Design review of the part shown in the three views and the two pictorial views. Dimensions are in mm from the part's minimum x, y and z. A direction names the side the tool comes from. Coordinates: 2 decimals unless noted, no trailing zeros. Order: outer loops, then holes, each group sorted by start corner. A loop starts at its lowest first (then second) coordinate and runs counter-clockwise, first axis right, second up. Notation, with made-up numbers: (26.25, 88) -> (75.25, 88) arc R36 ccw to (75.25, 127) -> close; hole circle Ø4 at (49.25, -1.5). An arc over 180 degrees is marked (long way). Answer as a JSON object with one key per item and string values. Group by question number.
1) Add section B-B, the plane z = 10.5. Write out the cut boundary in (x, y), then the cut area to 3 significant figures.
2) Add section D-D, the plane y = 40. Write out the cut boundary in (x, z), then the cut area to 3 significant figures.
3) Add section C-C, the plane z = 34. Write out the cut boundary in (x, y), then the cut area to 3 significant figures.
4) Machinability: for the marked faces 1 and 2, which of the approach directions +Z, -Z, +X, -X, +Y, -Y give a long, thin tool a straight path to every point of the face, cutting with its end or side? Answer none if there is none.
5) Wall thickness on L1, parallel to Y at x = 40, z = 2; L2, parallel to X at y = 21, z = 24; L3, parallel to Y at x = 28, z = 6.25: over which ranges is each line inside the solid? List them lowest first.
6) Draft analysis for pull direction X (two halves, no side actions). For the marked faces 3, 4, 5 and 6, state which applies: +X half, -X half, draft (parallel to the pull), parting line (faces both ways), or undercut.
7) For pin 1 (2 mm diameter, centred on y = 48, z = 22.5, fed in from -X); pin 2 (12 mm diameter, centred on x = 21.5, y = 25.5, fed in from +Z); pin 3 (11 mm diameter, centred on x = 36.5, z = 25, fed in from +Y), all flat-tipped, find the tip position at first contact; note any pin that passes through.
8) Add section A-A, the plane x = 78. Write out the cut boundary in (y, z), then the cut area to 3 significant figures.
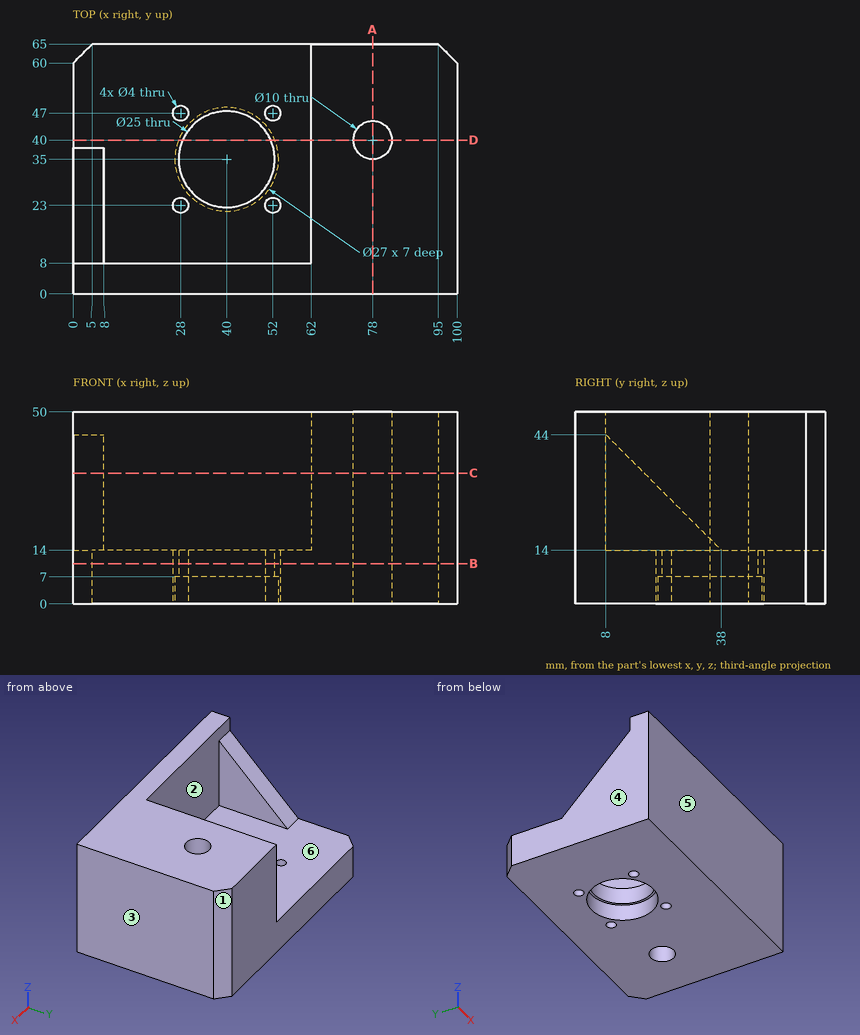
Output values:
{
 "1": {"outline": "(0, 0) -> (100, 0) -> (100, 60) -> (95, 65) -> (5, 65) -> (0, 60) -> close; hole circle Ø4 at (28, 23); hole circle Ø4 at (28, 47); hole circle Ø25 at (40, 35); hole circle Ø4 at (52, 23); hole circle Ø4 at (52, 47); hole circle Ø10 at (78, 40)", "area": "5,860 mm²"},
 "2": {"outline": "(0, 0) -> (27.46, 0) -> (27.46, 7) -> (28.54, 7) -> (28.54, 14) -> (0, 14) -> close; (51.46, 7) -> (52.54, 7) -> (52.54, 0) -> (73, 0) -> (73, 50) -> (62, 50) -> (62, 14) -> (51.46, 14) -> close; (83, 0) -> (100, 0) -> (100, 50) -> (83, 50) -> close", "area": "1,930 mm²"},
 "3": {"outline": "(0, 0) -> (100, 0) -> (100, 60) -> (95, 65) -> (62, 65) -> (62, 8) -> (8, 8) -> (8, 18) -> (0, 18) -> close; hole circle Ø10 at (78, 40)", "area": "2,950 mm²"},
 "4": {"face 1": "+Z, -Z, +X, +Y", "face 2": "+Z, +Y"},
 "5": {"L1": "y = 0 to 21.5, 48.5 to 65", "L2": "x = 0 to 8, 62 to 100", "L3": "y = 0 to 21, 25 to 28.82, 41.18 to 45, 49 to 65"},
 "6": {"face 3": "+X half", "face 4": "-X half", "face 5": "draft", "face 6": "undercut"},
 "7": {"pin 1": "stops at x = 62", "pin 2": "stops at z = 14", "pin 3": "stops at y = 8"},
 "8": {"outline": "(0, 0) -> (35, 0) -> (35, 50) -> (0, 50) -> close; (45, 0) -> (65, 0) -> (65, 50) -> (45, 50) -> close", "area": "2,750 mm²"}
}
